Read the model definition and answer for the solid it produces. Units are mm, in the model's axes. Give positions to 0.01 mm unless a question says otherwise; leave off trailing zeros. Order: outer loops, then holes, each group sorted by start corner. A loop starts at its lowest first (then second) coordinate and runs counter-clockwise, first axis right, second up.
Autodesk Inventor part; units mm, degrees
ref_plane "YZ Plane" through (0, 0, 0) normal (1, 0, 0) x (0, 1, 0)
ref_plane "XZ Plane" through (0, 0, 0) normal (0, 1, 0) x (-1, 0, 0)
ref_plane "XY Plane" through (0, 0, 0) normal (0, 0, 1) x (1, 0, 0)
sketch "Sketch1" plane through (0, 0, 0) normal (0, 0, 1) x (1, 0, 0)
  line L0 (0, 0) -> (25.4, 0)
  line L1 (25.4, 0) -> (25.4, 76.2)
  line L2 (25.4, 76.2) -> (0, 76.2)
  line L3 (0, 76.2) -> (0, 0)
  line L4 (0, 0) -> (6.35, 0)
  line L5 (6.35, 0) -> (6.35, 76.2) construction
  line L6 (6.35, 0) -> (25.4, 0)
  line L7 (15.875, 0) -> (15.875, 76.2) construction
  line L8 (15.875, 0) -> (15.875, 12.7) construction
  line L9 (15.875, 76.2) -> (15.875, 63.5) construction
  circle A0 centre (15.875, 12.7) radius 2.54
  circle A1 centre (15.875, 63.5) radius 2.54
  dimension "d0" = 25.4
  dimension "d1" = 76.2
  dimension "d2" = 6.35
  dimension "d3" = 12.7
  dimension "d4" = 12.7
  dimension "d5" = 5.08
extrude "Extrusion1" add sketch "Sketch1" along normal blind 15.24
properties part number "Beefy Spacer" material "Aluminum 6061"
1) Given pin 1 (10 mm diameter, centred on x = 14.5, y = 28.5, fed in from -Z), flat-ended and moving along its own axis, determine where the tip first touches the part or whether it passes through.
Final values:
pin 1: stops at z = 0
2) The part is cut by section C-C on y = 62. Determine the outline of the cut face in (x, z), and give its area (3 significant figures).
Final values:
outline: (0, 0) - (13.83, 0) - (13.83, 15.24) - (0, 15.24) - close; (17.92, 0) - (25.4, 0) - (25.4, 15.24) - (17.92, 15.24) - close
area: 325 mm2
3) For a pull along Y with two mould halves and no side action, classify faces 1 (the face through (18.221, 64.473, 7.513)), 2 (the face through (13, 39, 15.24)), 3 (the face through (13, 0, 8)), 4 (the face through (13, 76.2, 8)) as released by +Y, released by -Y, zero draft, split by the parting line, or undercut.
Final values:
face 1: undercut
face 2: zero draft
face 3: released by -Y
face 4: released by +Y
4) The part is cut by section B-B on x = 14. Determine the outline of the cut face in (y, z), and give its area (3 significant figures).
Final values:
outline: (0, 0) - (10.99, 0) - (10.99, 15.24) - (0, 15.24) - close; (14.41, 0) - (61.79, 0) - (61.79, 15.24) - (14.41, 15.24) - close; (65.21, 0) - (76.2, 0) - (76.2, 15.24) - (65.21, 15.24) - close
area: 1,060 mm2
5) The part is cut by section A-A on y = 12.7. Determine the outline of the cut face in (x, z) (3 decimals), and give its area (3 significant figures).
Final values:
outline: (0, 0) - (13.335, 0) - (13.335, 15.24) - (0, 15.24) - close; (18.415, 0) - (25.4, 0) - (25.4, 15.24) - (18.415, 15.24) - close
area: 310 mm2
6) Consider L1, parallel to Y at x = 17.75, z = 4.75; L2, parallel to Y at x = 14.25, z = 10.75; L3, parallel to X at y = 10.5, z = 13.5. Determine where each line is inside the solid, lowest interval first.
Final values:
L1: y = 0 to 10.99, 14.41 to 61.79, 65.21 to 76.2
L2: y = 0 to 10.75, 14.65 to 61.55, 65.45 to 76.2
L3: x = 0 to 14.61, 17.14 to 25.4
